Part model, mm, in its own coordinate system. A direction names the side the tool comes from. Round coordinates to 2 decimals unless told otherwise and drop trailing zeros. Loops run counter-clockwise (first coordinate to the right, second up) from the corner with the lowest first, then second, coordinate; pieces in that order, holes last. Notation, with made-up numbers: (79.25, 14.25) -> (125.25, 14.25) arc R29 cw to (125.25, 35.25) -> close; hole circle Ø11 at (46, -8.5). An arc over 180 degrees is marked (long way). Use a Markdown table: item, result. Add a question column.
Item 1: Which spindle directions (+Z, -Z, +X, -X, +Y, -Y) get a long thin tool onto all of the face, cutting with end or side? Do faces 1 (the face through (0, -7, 0)), 2 (the face through (-2.17, -9.76, 8.53)), 3 (the face through (2.1, -2.1, 17.3)). Say none if no direction does.
Item 2: Probe line 1 (Z direction, x = -7, y = -4.5); line 2 (X direction, y = -2.5, z = 17.5); line 3 (Z direction, x = -4.5, y = -2.5). List the from-to ranges inside material, lowest first. Write a range as [from, to].
Item 3: Flat gauge pins, fed straight in: pin 1 (6 mm diameter, centred on x = -4, y = -7.5, fed in from +Z); pin 2 (5 mm diameter, centred on y = 6, z = 29.5, fed in from +X); pin 3 (2 mm diameter, centred on x = -7.5, y = 0.5, fed in from -Z); pin 4 (2 mm diameter, centred on y = -6, z = 10.5, fed in from -X). Where does each tip first touch, or does it go through?
Item 4: Cut at A-A, the plane z = 5.5. List the corners of the cut face in (x, y), plus the area to 3 significant figures.
Item 5: Cut at C-C, the plane z = 26. List the corners of the cut face in (x, y), plus the area to 3 significant figures.
Item 6: Cut at B-B, the plane y = -6.5. List the corners of the cut face in (x, z).
```python
from build123d import *

# Parameters (mm, degrees)
ESQUISSE1_R        = 10
BOSS_EXTRU_1_DEPTH = 17.3
ESQUISSE2_R        = 2.75
BOSS_EXTRU_2_DEPTH = 28
ESQUISSE3_R        = 6
BOSS_EXTRU_3_DEPTH = 2.7
CONG_2_R           = 6


with BuildPart() as part:
    # Esquisse1 → Boss.-Extru.1 (new body)
    with BuildSketch(Plane.XY):
        Circle(ESQUISSE1_R)
    extrude(amount=BOSS_EXTRU_1_DEPTH)

    # Esquisse2 → Boss.-Extru.2 (add)
    with BuildSketch(Plane.XY.offset(17.3)):
        Circle(ESQUISSE2_R)
    extrude(amount=BOSS_EXTRU_2_DEPTH)

    # Esquisse3 → Boss.-Extru.3 (add)
    with BuildSketch(Plane(origin=(0, 0, 0), x_dir=(-1, 0, 0), z_dir=(0, 0, -1))):
        with Locations(Location((0, 0, 0), (0, 0, 180))):
            Circle(ESQUISSE3_R)
    extrude(amount=BOSS_EXTRU_3_DEPTH)

    # Congé2
    # the kernel refuses this fillet: 6 mm, written as the material it takes off along each edge
    with BuildSketch(Plane(origin=(0, 0, -2.7), x_dir=(1, 0, 0), z_dir=(0, 1, 0))) as cong_2_piece_1:
        with BuildLine():
            CenterArc((0.989012073, -6), CONG_2_R, 33.367012969, 56.632987031)
            Line((0.989012073, 0), (0.989012073, 0.12))
            Line((0.989012073, 0.12), (6, 0.12))
            Line((6, 0.12), (6.12, 0))
            ThreePointArc((6.12, 0), (6.12, -1.35), (6.100219759, -2.634))
            Line((6.100219759, -2.634), (6, -2.7))
        make_face()
    revolve(axis=Axis((0, 0, -2.7), (0, 0, -1)), mode=Mode.SUBTRACT)


solid = part.part
```
A:
| question | item | result |
|---|---|---|
| 1 | face 1 | -Z |
| 1 | face 2 | +Z, -Z |
| 1 | face 3 | +Z |
| 2 | line 1 | z = [0, 17.3] |
| 2 | line 2 | x = [-1.15, 1.15] |
| 2 | line 3 | z = [-1.02, 17.3] |
| 3 | pin 1 | stops at z = 17.3 |
| 3 | pin 2 | passes through |
| 3 | pin 3 | stops at z = 0 |
| 3 | pin 4 | stops at x = -8.66 |
| 4 | outline | circle Ø20 at (0, 0) |
| 4 | area | 314 mm^2 |
| 5 | outline | circle Ø5.5 at (0, 0) |
| 5 | area | 23.8 mm^2 |
| 6 | outline | (-7.6, 0) -> (7.6, 0) -> (7.6, 17.3) -> (-7.6, 17.3) -> close |
